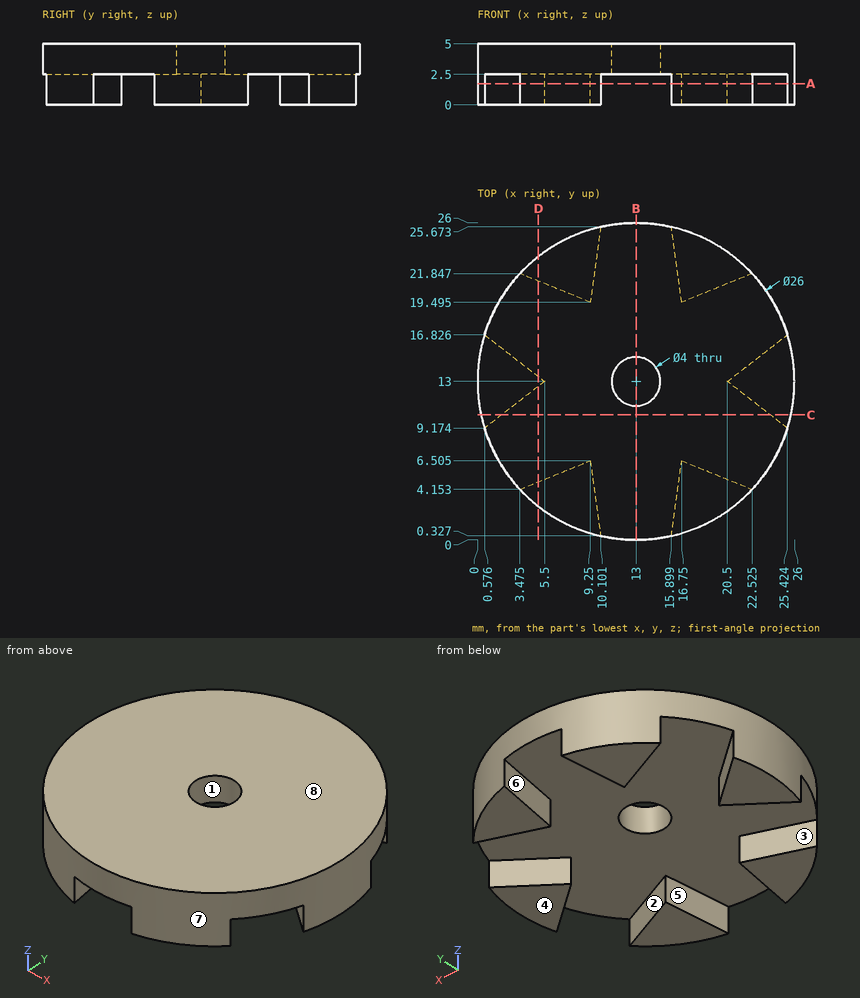
Can you work these out from the drawing? Everything is in mm from the part's minimum corner. A direction names the side the tool comes from. Give positions to 0.01 mm unless a question says otherwise; leave off trailing zeros. Order: outer loops, then holes, each group sorted by start corner. A loop starts at its lowest first (then second) coordinate and runs counter-clockwise, first axis right, second up.
1. For the marked faces 1, 2, 3, 4 and 5, which set-ups out of +Z, -Z, +X, -X, +Y, -Y let a thin tool reach every point of the face, with its end or its side?
2. Suppose I cut it at B-B (x = 13). List the corners of the cut face in (y, z) for me.
3. Suppose I cut it at C-C (y = 10.25). List the corners of the cut face in (x, z) for me.
4. I need wall thicknesses on L1, parallel to Y at x = 13, z = 3.15; L2, parallel to Z at x = 15.25, y = 8.25; L3, parallel to Y at x = 12.5, z = 3.15. Which ranges of each line are inside material? Lowest first, please.
5. Suppose I cut it at D-D (x = 5). List the corners of the cut face in (y, z) for me.
6. Suppose I cut it at A-A (z = 1.75). Give the number of separate pieces and of enclosed holes in the cut face, plus the area to 3 significant figures.
7. We'd pull the mould along Y, two halves only. Please class the marked faces 6, 7 and 8: pulls with the +Y half, pulls with the -Y half, needs draft (parallel to the pull), parting line crosses it, or undercut.
8. Will these pins go through, and if not, where does the flat tip stop? P1, Ø7.5, axis at x = 12.5, y = 11.5, coming from the -Z side; P2, Ø2, axis at y = 22, z = 4.5, coming from the +X side; P3, Ø2.5, axis at x = 13, y = 13, coming from the +Z side; P4, Ø6, axis at x = 21, y = 21, coming from the -Z side.
Solved:
1. face 1: +Z, -Z
1. face 2: -Z, +X
1. face 3: -Z, -X
1. face 4: -Z, +X, -X, +Y, -Y
1. face 5: -Z
2. outline: (0, 2.5) - (11, 2.5) - (11, 5) - (0, 5) - close; (15, 2.5) - (26, 2.5) - (26, 5) - (15, 5) - close
3. outline: (0.29, 0) - (1.96, 0) - (1.96, 2.5) - (24.04, 2.5) - (24.04, 0) - (25.71, 0) - (25.71, 5) - (0.29, 5) - close
4. L1: y = 0 to 11, 15 to 26
4. L2: z = 2.5 to 5
4. L3: y = 0.01 to 11.06, 14.94 to 25.99
5. outline: (2.75, 0) - (4.77, 0) - (4.77, 2.5) - (12.61, 2.5) - (12.61, 0) - (13.39, 0) - (13.39, 2.5) - (21.23, 2.5) - (21.23, 0) - (23.25, 0) - (23.25, 5) - (2.75, 5) - close
6. separate pieces: 6
6. enclosed holes: 0
6. area: 131 mm2
7. face 6: undercut
7. face 7: parting line crosses it
7. face 8: needs draft
8. P1: stops at z = 2.5
8. P2: stops at x = 23.25
8. P3: passes through
8. P4: stops at z = 0
